```python
from build123d import *

# Parameters (mm, degrees)
F0_W     = 114.3
F0_H     = 25.4
F1_DEPTH = 6.35
F2_W     = 114.3
F2_H     = 25.4
F3_DEPTH = 6.35
F4_W     = 114.3
F4_H     = 25.4
F5_DEPTH = 6.35
F6_W     = 114.3
F6_H     = 25.4
F7_DEPTH = 6.35
F9_DEPTH = 6.35


with BuildPart() as f1:
    # F0 (on Front) → F1 (new body)
    with BuildSketch(Plane.XZ):
        with Locations((57.15, 12.7)):
            Rectangle(F0_W, F0_H)
    extrude(amount=F1_DEPTH)

    # F2 (on face) → F3 (join)
    with BuildSketch(Plane(origin=(0, 0, 0), x_dir=(-1, 0, 0), z_dir=(0, 1, 0))):
        with Locations((18.810974, 12.7)):
            Rectangle(F2_W, F2_H)
    extrude(amount=F3_DEPTH)

    # F4 (on face) → F5 (join)
    with BuildSketch(Plane(origin=(0, 6.35, 0), x_dir=(-1, 0, 0), z_dir=(0, 1, 0))):
        with Locations((-57.389026, 12.7)):
            Rectangle(F4_W, F4_H)
    extrude(amount=F5_DEPTH)

    # F6 (on face) → F7 (join)
    with BuildSketch(Plane(origin=(0, 0, 0), x_dir=(-1, 0, 0), z_dir=(0, 1, 0))):
        with Locations((-133.469513, 12.7)):
            Rectangle(F6_W, F6_H)
    extrude(amount=F7_DEPTH)

    # F8 (on face) → F9 (join)
    with BuildSketch(Plane.XY.offset(25.4)):
        Polygon((-126.760974, 3.175), (-85.020583, 3.175), (-12.460974, 3.175), (-12.460974, 15.875), (-126.760974, 15.875), align=None)
        Polygon((-12.460974, 3.175), (-85.020583, 3.175), (-126.760974, 3.175), (-126.760974, -9.525), (-12.460974, -9.525), align=None)
    extrude(amount=F9_DEPTH)


solid = f1.part
```
Design review of the part built by this model. Coordinates are the model's own, in mm. A direction names the side the tool comes from. Coordinates: 2 decimals unless noted, no trailing zeros. Order: outer loops, then holes, each group sorted by start corner. A loop starts at its lowest first (then second) coordinate and runs counter-clockwise, first axis right, second up. Notation, with made-up numbers: M 63,-33 L 67,-33 A6 ccw 67,-24 Z; hole C -4,65 d9. An arc over 180 degrees is marked long. Answer as a JSON object with one key per item and string values. Group by question number.
1) Tool access review of faces 4 (the flat face through (-12.461, 3, 29)), 5 (the flat face through (-37, 0, 13)), 6 (the flat face through (-75.961, 3, 13)), 7 (the flat face through (0.239, 9, 13)): name each direction out of +Z, -Z, +X, -X, +Y, -Y from which nothing blocks a thin tool from reaching the whole face with its end or side.
2) Mouldability with a two-part tool opening along X and no side actions: class faces 1 (the flat face through (114.3, -3, 13)), 2 (the flat face through (153, 0, 13)), 3 (the flat face through (76.32, 3, 13)) as pulls with the +X half, pulls with the -X half, needs draft (parallel to the pull), parting line crosses it, or undercut.
3) Add section A-A, the plane y = -3.25. Write out the cut boundary in (x, z), then the cut area to 3 significant figures.
4) Add section B-B, the plane z = 21. Write out the cut boundary in (x, y).
5) For pin 1 (7 mm diameter, centred on y = 2, z = 17, fed in from -X); pin 2 (7.5 mm diameter, centred on x = 170.5, z = 14, fed in from -Y); pin 3 (3 mm diameter, centred on y = 9, z = 17, fed in from +X); pin 4 (10 mm diameter, centred on y = -4.5, z = 8, fed in from +X), all flat-tipped, find the tip position at first contact; note any pin that passes through.
6) Add section C-C, the plane x = -15.5. Write out the cut boundary in (y, z) (3 decimals), then the cut area to 3 significant figures.
7) Add section D-D, the plane x = 154.5. Write out the cut boundary in (y, z).
8) Wall thickness on L1, parallel to X at y = 2.5, z = 24; L2, parallel to X at y = -4.5, z = 10.5; L3, parallel to Y at x = 94.5, z = 14: over which ranges is each line inside the solid? List them lowest first.
Computed values:
{
 "1": {"face 4": "+Z, +X, +Y, -Y", "face 5": "-Z, -X, -Y", "face 6": "-Z, -X, +Y, -Y", "face 7": "+Z, -Z, -X, +Y"},
 "2": {"face 1": "pulls with the +X half", "face 2": "needs draft", "face 3": "undercut"},
 "3": {"outline": "M -126.76,25.4 L -12.46,25.4 L -12.46,31.75 L -126.76,31.75 Z; M 0,0 L 114.3,0 L 114.3,25.4 L 0,25.4 Z", "area": "3,630 mm^2"},
 "4": {"outline": "M -75.96,0 L 0,0 L 0,-6.35 L 114.3,-6.35 L 114.3,0 L 190.62,0 L 190.62,6.35 L 114.54,6.35 L 114.54,12.7 L 0.24,12.7 L 0.24,6.35 L -75.96,6.35 Z; hole M 38.34,0 L 76.32,0 L 76.32,6.35 L 38.34,6.35 Z"},
 "5": {"pin 1": "stops at x = -75.96", "pin 2": "stops at y = 0", "pin 3": "stops at x = 114.54", "pin 4": "stops at x = 190.62"},
 "6": {"outline": "M -9.525,25.4 L 0,25.4 L 0,0 L 6.35,0 L 6.35,25.4 L 15.875,25.4 L 15.875,31.75 L -9.525,31.75 Z", "area": "323 mm^2"},
 "7": {"outline": "M 0,0 L 6.35,0 L 6.35,25.4 L 0,25.4 Z"},
 "8": {"L1": "x = -75.96 to 38.34, 76.32 to 190.62", "L2": "x = 0 to 114.3", "L3": "y = -6.35 to 12.7"}
}
